Could you check a few things on this model? Use its own coordinates, in mm. Give positions to 0.01 mm unless a question says otherwise; leave off trailing zeros.
from build123d import *

# Parameters (mm, degrees)
F0_W     = 330.2
F0_H     = 215.9
F1_DEPTH = 12.7
F2_R     = 10.16
F3_R     = 10.16
F4_R     = 5.08
F5_W     = 15.24
F5_H     = 4.572
F6_DEPTH = 10.16
F7_W     = 11.379987
F7_H     = 5.284949
F8_DEPTH = 6.35


with BuildPart() as f1:
    # F0 (on Top) → F1 (new body)
    with BuildSketch(Plane.XY):
        Rectangle(F0_W, F0_H)
    extrude(amount=-F1_DEPTH)

    # F2
    f2_edges = [f1.edges().sort_by_distance(p)[0] for p in [
        (165.1, -107.95, -6.35),
    ]]
    fillet(f2_edges, radius=F2_R)

    # F3
    f3_edges = [f1.edges().sort_by_distance(p)[0] for p in [
        (-165.1, -107.95, -6.35),
    ]]
    fillet(f3_edges, radius=F3_R)

    # F4
    f4_edges = [f1.edges().sort_by_distance(p)[0] for p in [
        (0, -107.95, -12.7),
        (-162.124205, -104.974205, -12.7),
        (162.124205, -104.974205, -12.7),
        (-165.1, 5.08, -12.7),
        (165.1, 5.08, -12.7),
        (0, 107.95, -12.7),
    ]]
    fillet(f4_edges, radius=F4_R)

    # F5 (on face) → F6 (join)
    with BuildSketch(Plane.YZ.offset(165.1)):
        with Locations((97.510784, -5.334)):
            Rectangle(F5_W, F5_H)
    extrude(amount=-F6_DEPTH)

    # F7 (on face) → F8 (cut)
    with BuildSketch(Plane.YZ.offset(165.1)):
        with Locations((98.617143, -4.977525)):
            Rectangle(F7_W, F7_H)
    extrude(amount=-F8_DEPTH, mode=Mode.SUBTRACT)


solid = f1.part
Item 1: We'd pull the mould along Z, two halves only. Please class faces 1 (the cylindrical face through (162.045, -105.053, -3.863)), 2 (the flat face through (162, 99, -7.62)), 3 (the flat face through (-2, 1, -12.7)), 4 (the flat face through (162, 99, -2.335)): +Z half, -Z half, draft (parallel to the pull), parting line (faces both ways), or undercut.
Findings:
face 1: draft
face 2: undercut
face 3: -Z half
face 4: undercut
Item 2: Please list where these lines run through material, in increasing order: line 1 along Y through (x, z) = (30.5, -8.5); line 2 along X through (y, z) = (96, -8.75); line 3 along X through (y, z) = (-73.5, -7.75).
Findings:
line 1: y = -107.87 to 107.87
line 2: x = -164.97 to 164.97
line 3: x = -165.1 to 165.1
Item 3: For pin 1 (4 mm diameter, centred on x = 161.5, z = -6, fed in from -Y); pin 2 (2.5 mm diameter, centred on y = 100, z = -5.5, fed in from +X), each with a flat end and sliding along its axis, tell me the tip position at first contact or that it passes through.
Findings:
pin 1: stops at y = -106.87
pin 2: stops at x = 158.75
